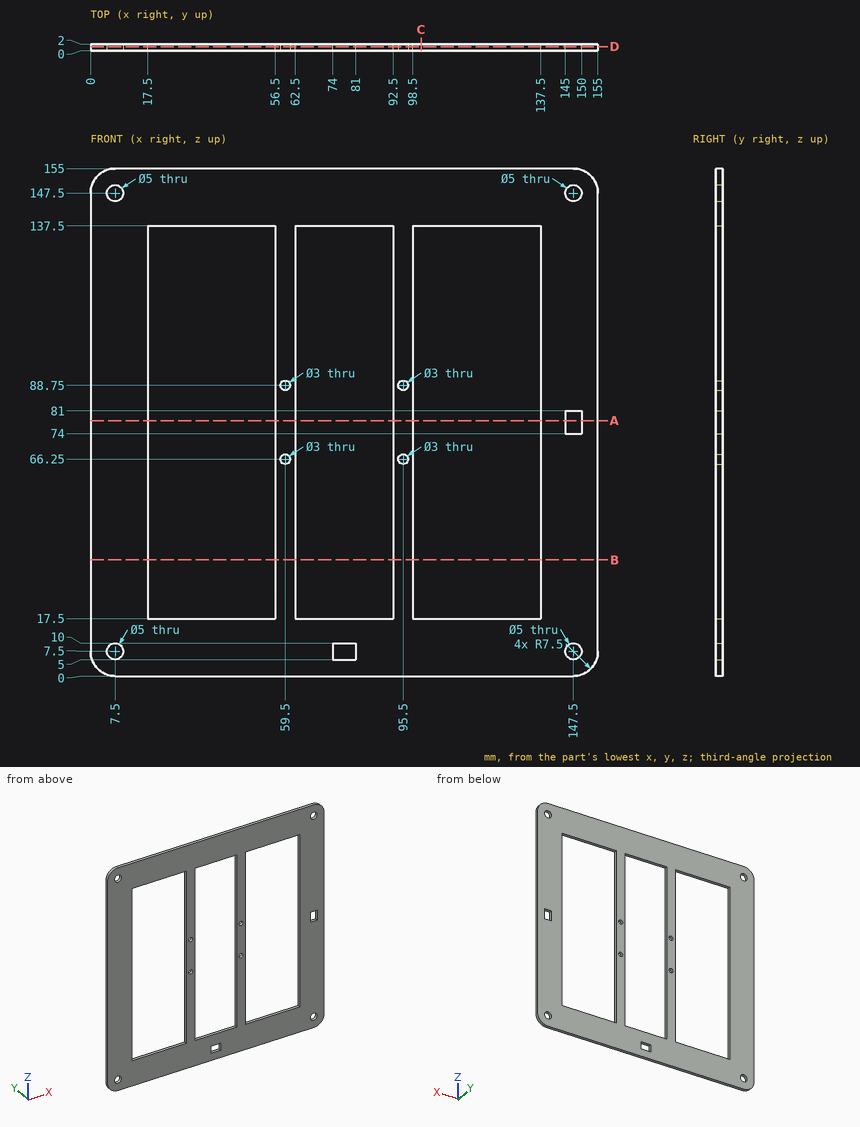
Here's the drawing with two shaded views (mm, measured from the low corner). I have some questions. Round coordinates to 2 decimals unless told otherwise and drop trailing zeros. Write each loop counter-clockwise with the first axis right and the second up, starting at its lowest first coordinate (ties: lowest second). Pieces come first, ordered by that corner, then holes.
(1) Suppose I cut it at B-B on z = 35.5. Write out the boundary of the cut face in (x, y), and give its area (3 significant figures).
Findings below:
outline: (0, 0) - (17.5, 0) - (17.5, 2) - (0, 2) - close; (56.5, 0) - (62.5, 0) - (62.5, 2) - (56.5, 2) - close; (92.5, 0) - (98.5, 0) - (98.5, 2) - (92.5, 2) - close; (137.5, 0) - (155, 0) - (155, 2) - (137.5, 2) - close
area: 94.0 mm2
(2) Suppose I cut it at A-A on z = 78. Write out the boundary of the cut face in (x, y).
Findings below:
outline: (0, 0) - (17.5, 0) - (17.5, 2) - (0, 2) - close; (56.5, 0) - (62.5, 0) - (62.5, 2) - (56.5, 2) - close; (92.5, 0) - (98.5, 0) - (98.5, 2) - (92.5, 2) - close; (137.5, 0) - (145, 0) - (145, 2) - (137.5, 2) - close; (150, 0) - (155, 0) - (155, 2) - (150, 2) - close
(3) If I drill on probe 1 along X at (y, z) = (1.4, 88.75); probe 2 along X at (y, z) = (1.45, 116.5); probe 3 along X at (y, z) = (1.5, 7.5), over which ranges is the centre line in solid material (lowest first)?
Findings below:
probe 1: x = 0 to 17.5, 56.5 to 58, 61 to 62.5, 92.5 to 94, 97 to 98.5, 137.5 to 155
probe 2: x = 0 to 17.5, 56.5 to 62.5, 92.5 to 98.5, 137.5 to 155
probe 3: x = 0 to 5, 10 to 74, 81 to 145, 150 to 155
(4) Suppose I cut it at D-D on y = 1.2. State how many separate pieces and enclosed holes the cut face has, and give its area (3 significant figures).
Findings below:
separate pieces: 1
enclosed holes: 13
area: 10,800 mm2
(5) Suppose I cut it at C-C on x = 101. Write out the boundary of the cut face in (y, z), and give its area (3 significant figures).
Findings below:
outline: (0, 0) - (2, 0) - (2, 17.5) - (0, 17.5) - close; (0, 137.5) - (2, 137.5) - (2, 155) - (0, 155) - close
area: 70.0 mm2
